```python
from build123d import *

# Parameters (mm, degrees)
F0_R        = 5.4864
F1_DEPTH    = 12.192
F3_DEPTH    = 19.05
F5_DEPTH    = 34.798
F6_R        = 10.033
F7_T4_DEPTH = 12.192
F7_T9_DEPTH = 12.192
F8_R        = 12.7
F10_DEPTH   = 25.4


# Not quite as in the source:
# - a fillet or chamfer that OpenCascade refuses, or shapes differently, is made with other operations: its cross-section is extruded or revolved along the edge and cut away or added


with BuildPart() as f1:
    # F0 (on Front) → F1 (new body)
    with BuildSketch(Plane.XZ):
        Polygon((-75.0316, 24.13), (-85.09, 24.13), (-85.09, -24.13), (-75.0316, -24.13), (-75.0316, -42.926), (77.216, -42.926), (77.216, 42.926), (-75.0316, 42.926), align=None)
        with Locations((-64.8462, -33.1216)):
            Circle(F0_R, mode=Mode.SUBTRACT)
        with Locations((64.9986, -33.1216)):
            Circle(F0_R, mode=Mode.SUBTRACT)
        with Locations((-64.8462, 32.8676)):
            Circle(F0_R, mode=Mode.SUBTRACT)
        with BuildLine():
            Line((35.941, -29.845), (-35.941, -29.845))
            ThreePointArc((-35.941, -29.845), (-65.786, 0), (-35.941, 29.845))
            Line((-35.941, 29.845), (35.941, 29.845))
            ThreePointArc((35.941, 29.845), (65.786, 0), (35.941, -29.845))
        make_face(mode=Mode.SUBTRACT)
        with Locations((64.9986, 32.8676)):
            Circle(F0_R, mode=Mode.SUBTRACT)
    extrude(amount=-F1_DEPTH)

    # F2 (on face) → F3 (join)
    with BuildSketch(Plane(origin=(0, 12.192, 0), x_dir=(-1, 0, 0), z_dir=(0, 1, 0))):
        with BuildLine():
            add(Edge.make_bspline(
                [(-61.0821252186, 18.9865), (-68.5165, 10.0378265977), (-68.5165, 0)],
                knots=[5.8130237676, 5.8130237676, 5.8130237676, 6.2831853072, 6.2831853072, 6.2831853072], degree=2, weights=[1, 0.9724955315, 1]))
            add(Edge.make_bspline(
                [(-68.5165, 0), (-68.5165, -10.0378265977), (-61.0821252186, -18.9865)],
                knots=[0, 0, 0, 0.4701615396, 0.4701615396, 0.4701615396], degree=2, weights=[1, 0.9724955315, 1]))
            add(Edge.make_bspline(
                [(-61.0821252186, -18.9865), (-9.5155823774, -81.056568289), (56.0204921364, -24.13)],
                knots=[0.4701615396, 0.4701615396, 0.4701615396, 2.5280622458, 2.5280622458, 2.5280622458], degree=2, weights=[1, 0.5157184224, 1]))
            add(Edge.make_bspline(
                [(56.0204921364, -24.13), (83.7998845283, 0), (56.0204921364, 24.13)],
                knots=[2.5280622458, 2.5280622458, 2.5280622458, 3.7551230613, 3.7551230613, 3.7551230613], degree=2, weights=[1, 0.8176204584, 1]))
            add(Edge.make_bspline(
                [(56.0204921364, 24.13), (-9.5155823774, 81.056568289), (-61.0821252186, 18.9865)],
                knots=[3.7551230613, 3.7551230613, 3.7551230613, 5.8130237676, 5.8130237676, 5.8130237676], degree=2, weights=[1, 0.5157184224, 1]))
        make_face()
        with BuildLine():
            ThreePointArc((35.941, 29.845), (65.786, 0), (35.941, -29.845))
            Line((35.941, -29.845), (-35.941, -29.845))
            ThreePointArc((-35.941, -29.845), (-65.786, 0), (-35.941, 29.845))
            Line((-35.941, 29.845), (35.941, 29.845))
        make_face(mode=Mode.SUBTRACT)
        with BuildLine():
            add(Edge.make_bspline(
                [(-68.5165, 0), (-68.5165, -10.0378265977), (-61.0821252186, -18.9865)],
                knots=[0, 0, 0, 0.4701615396, 0.4701615396, 0.4701615396], degree=2, weights=[1, 0.9724955315, 1]))
            add(Edge.make_bspline(
                [(-61.0821252186, 18.9865), (-68.5165, 10.0378265977), (-68.5165, 0)],
                knots=[5.8130237676, 5.8130237676, 5.8130237676, 6.2831853072, 6.2831853072, 6.2831853072], degree=2, weights=[1, 0.9724955315, 1]))
            Line((-61.0821252186, 18.9865), (-77.216, 18.9865))
            Line((-77.216, 18.9865), (-77.216, -18.9865))
            Line((-77.216, -18.9865), (-61.0821252186, -18.9865))
        make_face()
        with BuildLine():
            add(Edge.make_bspline(
                [(56.0204921364, -24.13), (83.7998845283, 0), (56.0204921364, 24.13)],
                knots=[2.5280622458, 2.5280622458, 2.5280622458, 3.7551230613, 3.7551230613, 3.7551230613], degree=2, weights=[1, 0.8176204584, 1]))
            Line((56.0204921364, -24.13), (85.09, -24.13))
            Line((85.09, -24.13), (85.09, 24.13))
            Line((85.09, 24.13), (56.0204921364, 24.13))
        make_face()
    extrude(amount=F3_DEPTH)

    # F4 (on face) → F5 (join)
    with BuildSketch(Plane(origin=(0, 31.242, 0), x_dir=(-1, 0, 0), z_dir=(0, 1, 0))):
        with BuildLine():
            add(Edge.make_bspline(
                [(-61.0821252186, 18.9865), (-68.5165, 10.0378265977), (-68.5165, 0)],
                knots=[5.8130237676, 5.8130237676, 5.8130237676, 6.2831853072, 6.2831853072, 6.2831853072], degree=2, weights=[1, 0.9724955315, 1]))
            add(Edge.make_bspline(
                [(-68.5165, 0), (-68.5165, -10.0378265977), (-61.0821252186, -18.9865)],
                knots=[0, 0, 0, 0.4701615396, 0.4701615396, 0.4701615396], degree=2, weights=[1, 0.9724955315, 1]))
            add(Edge.make_bspline(
                [(-61.0821252186, -18.9865), (-9.5155823774, -81.056568289), (56.0204921364, -24.13)],
                knots=[0.4701615396, 0.4701615396, 0.4701615396, 2.5280622458, 2.5280622458, 2.5280622458], degree=2, weights=[1, 0.5157184224, 1]))
            add(Edge.make_bspline(
                [(56.0204921364, -24.13), (83.7998845283, 0), (56.0204921364, 24.13)],
                knots=[2.5280622458, 2.5280622458, 2.5280622458, 3.7551230613, 3.7551230613, 3.7551230613], degree=2, weights=[1, 0.8176204584, 1]))
            add(Edge.make_bspline(
                [(56.0204921364, 24.13), (-9.5155823774, 81.056568289), (-61.0821252186, 18.9865)],
                knots=[3.7551230613, 3.7551230613, 3.7551230613, 5.8130237676, 5.8130237676, 5.8130237676], degree=2, weights=[1, 0.5157184224, 1]))
        make_face()
        with BuildLine():
            Line((-35.941, 29.845), (35.941, 29.845))
            ThreePointArc((35.941, 29.845), (65.786, 0), (35.941, -29.845))
            Line((35.941, -29.845), (-35.941, -29.845))
            ThreePointArc((-35.941, -29.845), (-65.786, 0), (-35.941, 29.845))
        make_face(mode=Mode.SUBTRACT)
    extrude(amount=F5_DEPTH)

    # F6
    f6_edges = [f1.edges().sort_by_distance(p)[0] for p in [
        (-75.0316, 6.096, 42.926),
        (77.216, 6.096, 42.926),
        (77.216, 6.096, -42.926),
        (-75.0316, 6.096, -42.926),
    ]]
    fillet(f6_edges, radius=F6_R)

    # F7: fillet of radius 10.16 on 2 edges, made by hand


with BuildPart() as f7_tool2:
    # F7_s3 → F7_t4 (new body)
    with BuildSketch(Plane.XZ):
        with BuildLine():
            ThreePointArc((-85.1432181398, -24.13), (-78.2119770428, -26.8614404589), (-75.0075612141, -33.5871069182))
            Line((-75.0075612141, -33.5871069182), (-73.9939955216, -33.5168176101))
            ThreePointArc((-73.9939955216, -33.5168176101), (-74.0156, -32.893), (-74.0156, -24.13))
            Line((-74.0156, -24.13), (-75.0316, -23.114))
            Line((-75.0316, -23.114), (-85.1432181398, -23.114))
            Line((-85.1432181398, -23.114), (-85.1432181398, -24.13))
        make_face()
    extrude(amount=-F7_T4_DEPTH)

    split(bisect_by=Plane.YZ.offset(-85.09), keep=Keep.TOP)


with BuildPart() as f1_1:
    add(f1.part)

    # F7_t1: union F7_tool2
    add(f7_tool2.part)


with BuildPart() as f7_tool7:
    # F7_s8 → F7_t9 (new body)
    with BuildSketch(Plane.XZ):
        with BuildLine():
            ThreePointArc((-75.0075612141, 33.5871069182), (-78.2119770428, 26.8614404589), (-85.1432181398, 24.13))
            Line((-85.1432181398, 24.13), (-85.1432181398, 23.114))
            Line((-85.1432181398, 23.114), (-75.0316, 23.114))
            Line((-75.0316, 23.114), (-74.0156, 24.13))
            ThreePointArc((-74.0156, 24.13), (-74.0156, 32.893), (-73.9939955216, 33.5168176101))
            Line((-73.9939955216, 33.5168176101), (-75.0075612141, 33.5871069182))
        make_face()
    extrude(amount=-F7_T9_DEPTH)

    split(bisect_by=Plane.YZ.offset(-85.09), keep=Keep.TOP)


with BuildPart() as f1_2:
    add(f1_1.part)

    # F7_t6: union F7_tool7
    add(f7_tool7.part)

    # F8 (call 1 of 4: OpenCascade refuses the feature's edges together)
    f8_edges = [f1_2.edges().sort_by_distance(p)[0] for p in [
        (-56.020492, 21.717, 24.13),
    ]]
    fillet(f8_edges, radius=F8_R)

    # F8#3 (call 2 of 4)
    f8_3_edges = [f1_2.edges().sort_by_distance(p)[0] for p in [
        (61.082125, 21.717, -18.9865),
    ]]
    fillet(f8_3_edges, radius=F8_R)

    # F8#4 (call 3 of 4)
    f8_4_edges = [f1_2.edges().sort_by_distance(p)[0] for p in [
        (-56.020492, 21.717, -24.13),
    ]]
    fillet(f8_4_edges, radius=F8_R)

    # F8#2 (call 4 of 4)
    f8_2_edges = [f1_2.edges().sort_by_distance(p)[0] for p in [
        (61.082125, 21.717, 18.9865),
    ]]
    fillet(f8_2_edges, radius=F8_R)

    # F9 (on face) → F10 (cut)
    with BuildSketch(Plane.XZ):
        with BuildLine():
            ThreePointArc((22.225, -38.9382), (24.765, -36.3982), (22.225, -33.8582))
            Line((22.225, -33.8582), (-22.225, -33.8582))
            ThreePointArc((-22.225, -33.8582), (-24.765, -36.3982), (-22.225, -38.9382))
            Line((-22.225, -38.9382), (22.225, -38.9382))
        make_face()
    extrude(amount=-F10_DEPTH, mode=Mode.SUBTRACT)


solid = f1_2.part
```
Design review of the part built by this model. Coordinates are the model's own, in mm. A direction names the side the tool comes from. Coordinates: 2 decimals unless noted, no trailing zeros. Loops run counter-clockwise (first coordinate to the right, second up) from the corner with the lowest first, then second, coordinate; pieces in that order, holes last. Notation, with made-up numbers: (73, 22) - (114, 22) arc R21 cw to (114, 30) - close; hole circle Ø6 at (74.25, -31). An arc over 180 degrees is marked (long way). Use CSV: the item, a comma, the result in double quotes. Start each with the question number.
1) Consider section A-A on y = 6.5. Write out the cut boundary in (x, z) (3 decimals), then the cut area to 3 significant figures.
2) Tool access review of faces 5 (the flat face through (4, 66.04, 30)), 6 (the flat face through (72, 22, -18.986)), 7 (the flat face through (72, 22, 18.986)), 8 (the flat face through (1, 33, 29.845)), 9 (the flat face through (-73, 22, -24.13)): name each direction out of +Z, -Z, +X, -X, +Y, -Y from which nothing blocks a thin tool from reaching the whole face with its end or side.
3) Wall thickness on L1, parallel to Z at x = 4, y = 14.5 (3 decimals); L2, parallel to Y at x = -72, z = 8; L3, parallel to X at y = 54, z = -2.5: over which ranges is each line inside the solid? List them lowest first. Write a range as from..to.
4) For pin 1 Ø21 at (x, y) = (-69, 23) entering from -Z; pin 2 Ø11.5 at (x, y) = (69.5, 25) entering from +Z; pin 3 Ø5.5 at (x, y) = (73, 22) entering from -Z, all flat-tipped, find the tip position at first contact; note any pin that passes through.
5) Consider section B-B on y = 17. Give the number of separate pieces and of enclosed holes in the cut face, then the cut area to 3 significant figures.
6) The part is to be moulded in two halves that separate along X. For faces 1 (the flat face through (13.7, 12.192, 41.3)), 2 (the cylindrical face through (60.645, 6.011, -36.46)), 3 (the flat face through (-1, 33, -29.845)), 4 (the cylindrical face through (-78.27, 6.01, -26.81)), say which applies: +X half, -X half, draft (parallel to the pull), parting line (faces both ways), or undercut.
Geometry says:
1,outline,"(-85.09, -24.13) arc R10.16 cw to (-75.008, -33.587) arc R10.033 ccw to (-64.999, -42.926) - (67.183, -42.926) arc R10.033 ccw to (77.216, -32.893) - (77.216, 32.893) arc R10.033 ccw to (67.183, 42.926) - (-64.999, 42.926) arc R10.033 ccw to (-75.008, 33.587) arc R10.16 cw to (-85.09, 24.13) - close; hole circle Ø10.973 at (-64.846, -33.122); hole circle Ø10.973 at (-64.846, 32.868); hole (-35.941, -29.845) - (35.941, -29.845) arc R29.845 ccw to (35.941, 29.845) - (-35.941, 29.845) arc R29.845 ccw to start; hole (-22.225, -38.938) - (22.225, -38.938) arc R2.54 ccw to (22.225, -33.858) - (-22.225, -33.858) arc R2.54 ccw to start; hole circle Ø10.973 at (64.999, -33.122); hole circle Ø10.973 at (64.999, 32.868)"
1,area,"5,800 mm^2"
2,face 5,"+Z, -Z, +X, -X, +Y"
2,face 6,"-Z, +X, +Y"
2,face 7,"+Z, +X, +Y"
2,face 8,"+Y, -Y"
2,face 9,"-Z, -X, +Y"
3,L1,"-41.839..-38.938, -33.858..-29.845, 29.845..41.839"
3,L2,"0..31.24"
3,L3,"-68.39..-65.68, 65.68..68.39"
4,pin 1,"z = -24.28"
4,pin 2,"z = 19.3"
4,pin 3,"z = -18.99"
5,separate pieces,"1"
5,enclosed holes,"2"
5,area,"3,110 mm^2"
6,face 1,"draft"
6,face 2,"undercut"
6,face 3,"undercut"
6,face 4,"-X half"
